Autodesk Inventor part; units mm, degrees
ref_plane "YZ Plane" through (0, 0, 0) normal (1, 0, 0) x (0, 1, 0)
ref_plane "XZ Plane" through (0, 0, 0) normal (0, 1, 0) x (-1, 0, 0)
ref_plane "XY Plane" through (0, 0, 0) normal (0, 0, 1) x (1, 0, 0)
sketch "스케치1" plane through (0, 0, 0) normal (0, 1, 0) x (-1, 0, 0)
  line L0 (74, 43) -> (-216, 43)
  line L1 (-216, 43) -> (-216, 76)
  line L2 (-216, 76) -> (74, 76)
  line L3 (74, 76) -> (74, 43)
  point P0 (0, 0)
  dimension "d0" = 290
  dimension "d1" = 33
extrude "돌출1" add sketch "스케치1" along normal blind 2
sketch "스케치2" plane through (0, 0, 0) normal (0, -1, 0) x (1, 0, 0)
  line L0 (216, 43) -> (-74, 43)
  line L1 (-74, 76) -> (216, 76)
  line L2 (173, 43) -> (167.8, 43)
  line L3 (167.8, 43) -> (167.8, 76)
  line L4 (167.8, 76) -> (173, 76)
  line L5 (173, 76) -> (173, 43)
  line L6 (216, 43) -> (216, 76)
  line L7 (216, 76) -> (-74, 76)
  line L8 (-74, 43) -> (216, 43)
  line L9 (-31, 76) -> (-25.8, 76)
  line L10 (-25.8, 76) -> (-25.8, 43)
  line L11 (-25.8, 43) -> (-31, 43)
  line L12 (-31, 43) -> (-31, 76)
  line L13 (-74, 76) -> (-74, 43)
  point P0 (0, 0)
  dimension "d4" = 5.2
  dimension "d5" = 43
  dimension "d6" = 5.2
  dimension "d7" = 43
extrude "돌출2" cut sketch "스케치2" against normal blind 1 contours L0 L3 L1 L5 | L0 L12 L1 L10
sketch "스케치3" plane through (0, 0, 0) normal (0, -1, 0) x (1, 0, 0)
  line L0 (173, 76) -> (173, 43)
  line L1 (173, 43) -> (216, 43)
  line L2 (216, 43) -> (216, 76)
  line L3 (216, 76) -> (173, 76)
  line L4 (-31, 43) -> (-31, 76)
  line L5 (-31, 76) -> (-74, 76)
  line L6 (-74, 76) -> (-74, 43)
  line L7 (-74, 43) -> (-31, 43)
  line L8 (215, 43) -> (215, 76)
  line L9 (-74, 76) -> (216, 76)
  line L10 (209.6, 43) -> (209.6, 76)
  line L11 (-74, 43) -> (-31, 43)
  line L12 (-73, 43) -> (-73, 76)
  line L13 (-67.6, 43) -> (-67.6, 76)
  line L14 (-31, 76) -> (-74, 76)
  point P0 (0, 0)
  dimension "d10" = 1
  dimension "d11" = 5.4
  dimension "d12" = 1
  dimension "d13" = 5.4
extrude "돌출3" cut sketch "스케치3" against normal blind 1 contours L3 L8 L1 L10 | L13 L7 L12 L5
properties part number "앞판_밑" material "알루미늄 6061"
Build history of the part. All positions in model axes, mm. A direction names the side the tool comes from. Round coordinates to 2 decimals unless told otherwise and drop trailing zeros. Order: outer loops, then holes, each group sorted by start corner. A loop starts at its lowest first (then second) coordinate and runs counter-clockwise, first axis right, second up. Notation, with made-up numbers: (9.25, 73.25) -> (36.25, 73.25) arc R24 cw to (36.25, 111.25) -> close; hole circle Ø2 at (76, -26). An arc over 180 degrees is marked (long way). Answer in a Markdown table with one row per item.
1) Which spindle directions (+Z, -Z, +X, -X, +Y, -Y) get a long thin tool onto all of the face, cutting with end or side? Do faces 4 (the flat face through (-28, 1, 60)), 5 (the flat face through (-49, 0, 60)). Say none if no direction does.
Values:
| item | result |
|---|---|
| face 4 | +Z, -Z, -Y |
| face 5 | +Z, -Z, +X, -X, -Y |
2) Band-saw the part on A-A on y = 0.45. Give the cut face in (x, z).
Values:
| item | result |
|---|---|
| outline | (-74, 43) -> (-73, 43) -> (-73, 76) -> (-74, 76) -> close; (-67.6, 43) -> (-31, 43) -> (-31, 76) -> (-67.6, 76) -> close; (-25.8, 43) -> (167.8, 43) -> (167.8, 76) -> (-25.8, 76) -> close; (173, 43) -> (209.6, 43) -> (209.6, 76) -> (173, 76) -> close; (215, 43) -> (216, 43) -> (216, 76) -> (215, 76) -> close |
3) Wall check: L1, parallel to X at y = 0.5, z = 74.5; L2, parallel to Y at x = 170, z = 68. Give the ranges that are in metal, low to high.
Values:
| item | result |
|---|---|
| L1 | -74 to -73, -67.6 to -31, -25.8 to 167.8, 173 to 209.6, 215 to 216 |
| L2 | 1 to 2 |
4) Pin check, flat tips, straight feed: P1, Ø4, axis at x = 170, z = 65, coming from the -Y side; P2, Ø1.5, axis at x = 135.5, z = 57, coming from the -Y side. Stop position of each tip, or through.
Values:
| item | result |
|---|---|
| P1 | y = 1 |
| P2 | y = 0 |
5) Mould opens along X. For faces 1 (the flat face through (192, 0, 60)), 2 (the flat face through (212, 1, 60)), 3 (the flat face through (-70, 1, 60)) say: released by +X, released by -X, zero draft, split by the parting line, or undercut.
Values:
| item | result |
|---|---|
| face 1 | zero draft |
| face 2 | undercut |
| face 3 | undercut |
6) Band-saw the part on B-B on z = 58. Give the cut face in (x, y), and give its area (3 significant figures).
Values:
| item | result |
|---|---|
| outline | (-74, 0) -> (-73, 0) -> (-73, 1) -> (-67.6, 1) -> (-67.6, 0) -> (-31, 0) -> (-31, 1) -> (-25.8, 1) -> (-25.8, 0) -> (167.8, 0) -> (167.8, 1) -> (173, 1) -> (173, 0) -> (209.6, 0) -> (209.6, 1) -> (215, 1) -> (215, 0) -> (216, 0) -> (216, 2) -> (-74, 2) -> close |
| area | 559 mm2 |
